Design review of the part built by this model. Coordinates are the model's own, in mm. Face numbers are marked on the shaded views. Coordinates: 2 decimals unless noted, no trailing zeros. Write each loop counter-clockwise with the first axis right and the second up, starting at its lowest first coordinate (ties: lowest second). Pieces come first, ordered by that corner, then holes. Notation, with made-up numbers: (-29.5, 41) - (-3.5, 41) arc R26 cw to (-3.5, 56) - close; hole circle Ø6 at (14.25, -11). An arc over 180 degrees is marked (long way). Use a Markdown table: item, result.
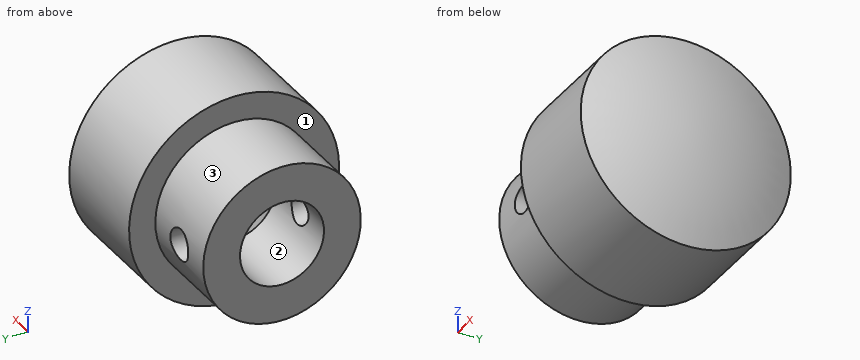
from build123d import *

# Parameters (mm, degrees)
F_8_0MM_1_D     = 8
F_8_0MM_1_DEPTH = 8
F_8_0MM_1_TIP   = 2.403442476


with BuildPart() as part:
    # 草图1 → 旋转1 (revolve)
    with BuildSketch(Plane.XY, mode=Mode.PRIVATE) as revolve_1_sk:
        with BuildLine():
            Line((0, 0), (0, 7.5))
            Line((0, 7.5), (8, 7.5))
            Line((8, 7.5), (8, 10))
            Line((8, 10), (18, 10))
            ThreePointArc((18, 10), (19.559779348, 5.107741092), (20.087121525, 0))
            Line((20.087121525, 0), (0, 0))
        make_face()
    revolve(revolve_1_sk.sketch.rotate(Axis((0, 0, 0), (1, 0, 0)), 90), axis=Axis((0, 0, 0), (1, 0, 0)))

    # Ø8.0mm 暗销孔1
    with Locations(Plane.ZY):
        with Locations((0, 0)):
            Hole(F_8_0MM_1_D / 2, depth=F_8_0MM_1_DEPTH)
            with Locations((0, 0, -(F_8_0MM_1_DEPTH + F_8_0MM_1_TIP / 2))):  # 118° drill point
                Cone(0, F_8_0MM_1_D / 2, F_8_0MM_1_TIP, mode=Mode.SUBTRACT)

    # 草图4 → 切除-旋转1 (revolve, cut)
    with BuildSketch(Plane.XY, mode=Mode.PRIVATE) as cut_revolve_1_sk:
        Polygon((4, -8.895136949), (5.4, -8.895136949), (5.5, 8.719380104), (4, 8.719380104), align=None)
    revolve(cut_revolve_1_sk.sketch.rotate(Axis((4, 18.564015212, 0), (0, -1, 0)), 226.690648884), axis=Axis((4, 18.564015212, 0), (0, -1, 0)), mode=Mode.SUBTRACT)


solid = part.part
(1) Draft analysis for pull direction Z (two halves, no side actions). For the marked faces 1, 2 and 3, state which applies: +Z half, -Z half, draft (parallel to the pull), parting line (faces both ways), or undercut.
Determined:
| item | result |
|---|---|
| face 1 | draft |
| face 2 | undercut |
| face 3 | parting line |
(2) For pin 1 (1.5 mm diameter, centred on x = 12, y = 7.5, fed in from -Z); pin 2 (1.5 mm diameter, centred on x = 13, y = -8, fed in from -Z); pin 3 (10 mm diameter, centred on x = 12.5, z = 6, fed in from -Y), all flat-tipped, find the tip position at first contact; note any pin that passes through.
Determined:
| item | result |
|---|---|
| pin 1 | z = -7.38 |
| pin 2 | z = -6.89 |
| pin 3 | y = -9.95 |
(3) Take a section at C-C on x = 11.25. Write out the cut boundary in (y, z).
Determined:
| item | result |
|---|---|
| outline | circle Ø20 at (0, 0) |
(4) For L1, parallel to Z at x = 13.25, y = -0.25; L2, parallel to Z at x = 9.5, y = -0.25; L3, parallel to Y at x = 10, z = 2.5, list the stretches that pass through material, from the lowest coordinate up. Write a range as from..to.
Determined:
| item | result |
|---|---|
| L1 | -10..10 |
| L2 | -10..-1.48, 1.48..10 |
| L3 | -9.68..9.68 |
(5) Take a section at D-D on y = -5.25. Write out the cut boundary in (x, z), and give its area (3 significant figures).
Determined:
| item | result |
|---|---|
| outline | (0, -5.36) - (8, -5.36) - (8, -8.51) - (18, -8.51) arc R24.44 ccw to (18, 8.51) - (8, 8.51) - (8, 5.36) - (0, 5.36) - close; hole circle Ø2.84 at (4, 0) |
| area | 267 mm2 |
(6) Take a section at A-A on y = 5.5. Write out the cut boundary in (x, z) (1 decimal), and give its area (3 significant figures).
Determined:
| item | result |
|---|---|
| outline | (0, -5.1) - (8, -5.1) - (8, -8.4) - (18, -8.4) arc R24.4 ccw to (18, 8.4) - (8, 8.4) - (8, 5.1) - (0, 5.1) - close; hole circle Ø3 at (4, 0) |
| area | 258 mm2 |
(7) Take a section at B-B on x = 1.75. Write out the cut boundary in (y, z), and give its area (3 significant figures).
Determined:
| item | result |
|---|---|
| outline | circle Ø15 at (0, 0); hole circle Ø8 at (0, 0) |
| area | 126 mm2 |
